Geometry check sheet. Reference: the model listing, model coordinates, mm. A direction names the side the tool comes from. Round coordinates to 2 decimals unless told otherwise and drop trailing zeros. Order: outer loops, then holes, each group sorted by start corner. A loop starts at its lowest first (then second) coordinate and runs counter-clockwise, first axis right, second up. Notation, with made-up numbers: M 12.5,28 L 22.5,28 A26 cw 22.5,66 Z; hole C -37,14 d9. An arc over 180 degrees is marked long. Answer as a JSON object with one key per item and string values. Group by question number.
```python
from build123d import *

# Parameters (mm, degrees)
F0_W     = 30
F0_H     = 10
F1_DEPTH = 1
F2_R     = 1
F3_DEPTH = 0.75


# Not quite as in the source:
# - a feature of the source that left no trace in its solid (it failed there, or was rolled back) is left out


with BuildPart() as f1:
    # F0 (on Top) → F1 (new body)
    with BuildSketch(Plane.XY):
        with Locations((0.392307792, 0)):
            Rectangle(F0_W, F0_H)
    extrude(amount=F1_DEPTH)

    # F2 (on Right) → F3 (join, symmetric)
    with BuildSketch(Plane.YZ):
        with BuildLine():
            Line((-5, 1), (5, 1))
            Line((5, 1), (5, 3.3628055826))
            Line((5, 3.3628055826), (-6.0430504382, 22.7664429694))
            Line((-6.0430504382, 22.7664429694), (-13.9894526005, 22.7664429694))
            ThreePointArc((-13.9894526005, 22.7664429694), (-15.4036661629, 22.1806565318), (-15.9894526005, 20.7664429694))
            Line((-15.9894526005, 20.7664429694), (-15.9894526005, 12.5754568726))
            Line((-15.9894526005, 12.5754568726), (-10.9724997157, 3.7602173598))
            Line((-10.9724997157, 3.7602173598), (-4.9831885844, 3.7602173598))
            Line((-4.9831885844, 3.7602173598), (-5, 1))
        make_face()
        with Locations((-12.1576432139, 18.2824078947)):
            Circle(F2_R, mode=Mode.SUBTRACT)
    extrude(amount=F3_DEPTH, both=True)


solid = f1.part
```
1) Go/stop test with flat-tipped pins: P1, Ø1, axis at y = -4, z = 6.5, coming from the -X side; P2, Ø1.5, axis at y = -2, z = 14, coming from the +X side; P3, Ø1.5, axis at x = -2.5, y = -9, coming from the +Z side; P4, Ø3, axis at x = -10.5, y = 1, coming from the +Z side. Record where each tip stops, or that it passes through.
2) Thickness scan on line 1 along Z through (x, y) = (-8.5, 2.25); line 2 along X through (y, z) = (-8, 7); line 3 along Y through (x, z) = (-0.25, 5). Record the ranges inside material, lowest first. Write a range as [from, to].
3) Sectioned sample at A-A (y = -4). Record the boundary of the cut face in (x, z).
4) Sectioned sample at B-B (z = 18.75). Record the boundary of the cut face in (x, y).
5) Sectioned sample at C-C (x = 10). Record the boundary of the cut face in (y, z), then the cut area to 3 significant figures.
6) Set-up check for faces 4 (the flat face through (0.75, -8, 12)), 5 (the flat face through (0, -13.5, 8.2)), 6 (the flat face through (-8, 0, 1)): record each of +Z, -Z, +X, -X, +Y, -Y from which the full face is reachable in a straight line by a thin tool's end or side.
7) Sectioned sample at D-D (y = 1). Record the boundary of the cut face in (x, z), then the cut area to 3 significant figures.
8) Release check for a two-part mould opening along Z. For faces 1 (the flat face through (0, -10, 22.766)), 2 (the cylindrical face through (-0.01, -11.62, 19.126)), 3 (the flat face through (0, -15.989, 17)) record: +Z half, -Z half, draft (parallel to the pull), parting line (faces both ways), or undercut.
Final values:
{
 "1": {"P1": "stops at x = -0.75", "P2": "stops at x = 0.75", "P3": "passes through", "P4": "stops at z = 1"},
 "2": {"line 1": "z = [0, 1]", "line 2": "x = [-0.75, 0.75]", "line 3": "y = [-11.68, 4.07]"},
 "3": {"outline": "M -14.61,0 L 15.39,0 L 15.39,1 L 0.75,1 L 0.75,19.18 L -0.75,19.18 L -0.75,1 L -14.61,1 Z"},
 "4": {"outline": "M -0.75,-15.99 L 0.75,-15.99 L 0.75,-13.04 L -0.75,-13.04 Z; M -0.75,-11.27 L 0.75,-11.27 L 0.75,-3.76 L -0.75,-3.76 Z"},
 "5": {"outline": "M -5,0 L 5,0 L 5,1 L -5,1 Z", "area": "10.0 mm^2"},
 "6": {"face 4": "+Z, +X, +Y, -Y", "face 5": "-Z, +X, -X, -Y", "face 6": "+Z, -X, +Y, -Y"},
 "7": {"outline": "M -14.61,0 L 15.39,0 L 15.39,1 L 0.75,1 L 0.75,10.39 L -0.75,10.39 L -0.75,1 L -14.61,1 Z", "area": "44.1 mm^2"},
 "8": {"face 1": "+Z half", "face 2": "undercut", "face 3": "draft"}
}
